Part model, mm, in its own coordinate system. Face numbers are marked on the shaded views. A direction names the side the tool comes from. Round coordinates to 2 decimals unless told otherwise and drop trailing zeros. Loops run counter-clockwise (first coordinate to the right, second up) from the corner with the lowest first, then second, coordinate; pieces in that order, holes last.
(1) Probe probe 1 along Z at (x, y) = (-9, -0.25); probe 2 along Y at (x, z) = (2.5, -7.5); probe 3 along X at (y, z) = (5.5, 7.5) (3 decimals). List the from-to ranges inside material, lowest first.
(2) Tool access for the marked faces 4, 5 and 6: list every direction of +Z, -Z, +X, -X, +Y, -Y with a clear straight run to the whole face (end or side of a thin tool).
(3) Flat gauge pins, fed straight in: pin 1 (1 mm diameter, centred on x = -2, z = -5, fed in from -Y); pin 2 (1.2 mm diameter, centred on x = -9.5, y = 0, fed in from -Z); pin 3 (3 mm diameter, centred on y = 2, z = -13, fed in from -X) (3 decimals). Where does each tip first touch, or does it go through?
(4) Cut at D-D on y = 4. List the corners of the cut face in (x, z) (3 decimals).
(5) Cut at B-B on x = 0. List the corners of the cut face in (y, z), then the cut area to 3 significant figures.
(6) Cut at C-C on z = -3.5. List the corners of the cut face in (x, y) (3 decimals), then the cut area to 3 significant figures.
(7) Mould opens along X. For the marked faces 1, 2 and 3 say: +X half, -X half, draft (parallel to the pull), parting line (faces both ways), or undercut.
(8) Cut at A-A on y = 5.5. List the corners of the cut face in (x, z) (3 decimals), then the cut area to 3 significant figures.
from build123d import *

# Parameters (mm, degrees)
EXTRUDE_1_DEPTH = 1.5
EXTRUDE_2_DEPTH = 3.175
SKETCH_9_R      = 2.3
EXTRUDE_3_DEPTH = 2


with BuildPart() as part:
    # 草图1 → 凸台-拉伸1 (new, symmetric)
    with BuildSketch(Plane(origin=(0, 0, 0), x_dir=(1, 0, 0), z_dir=(0, 1, 0))):
        with BuildLine():
            Line((-13, 2.1), (-13, -2.1))
            ThreePointArc((-13, -2.1), (-12.707106781, -2.807106781), (-12, -3.1))
            Line((-12, -3.1), (-6.4, -3.1))
            ThreePointArc((-6.4, -3.1), (-6.329289322, -3.070710678), (-6.3, -3))
            Line((-6.3, -3), (-6.3, -2.9))
            ThreePointArc((-6.3, -2.9), (-6.270710678, -2.829289322), (-6.2, -2.8))
            Line((-6.2, -2.8), (6.2, -2.8))
            ThreePointArc((6.2, -2.8), (6.270710678, -2.829289322), (6.3, -2.9))
            Line((6.3, -2.9), (6.3, -3))
            ThreePointArc((6.3, -3), (6.329289322, -3.070710678), (6.4, -3.1))
            Line((6.4, -3.1), (12, -3.1))
            ThreePointArc((12, -3.1), (12.707106781, -2.807106781), (13, -2.1))
            Line((13, -2.1), (13, 2.1))
            ThreePointArc((13, 2.1), (12.707106781, 2.807106781), (12, 3.1))
            Line((12, 3.1), (-12, 3.1))
            ThreePointArc((-12, 3.1), (-12.707106781, 2.807106781), (-13, 2.1))
        make_face()
        with BuildLine():
            Line((10.05, 1.65), (8.95, 1.65))
            ThreePointArc((8.95, 1.65), (7.81862915, 1.18137085), (7.35, 0.05))
            Line((7.35, 0.05), (7.35, -0.05))
            ThreePointArc((7.35, -0.05), (7.81862915, -1.18137085), (8.95, -1.65))
            Line((8.95, -1.65), (10.05, -1.65))
            ThreePointArc((10.05, -1.65), (11.18137085, -1.18137085), (11.65, -0.05))
            Line((11.65, -0.05), (11.65, 0.05))
            ThreePointArc((11.65, 0.05), (11.18137085, 1.18137085), (10.05, 1.65))
        make_face(mode=Mode.SUBTRACT)
        with BuildLine():
            Line((-10.05, 1.65), (-8.95, 1.65))
            ThreePointArc((-8.95, 1.65), (-7.81862915, 1.18137085), (-7.35, 0.05))
            Line((-7.35, 0.05), (-7.35, -0.05))
            ThreePointArc((-7.35, -0.05), (-7.81862915, -1.18137085), (-8.95, -1.65))
            Line((-8.95, -1.65), (-10.05, -1.65))
            ThreePointArc((-10.05, -1.65), (-11.18137085, -1.18137085), (-11.65, -0.05))
            Line((-11.65, -0.05), (-11.65, 0.05))
            ThreePointArc((-11.65, 0.05), (-11.18137085, 1.18137085), (-10.05, 1.65))
        make_face(mode=Mode.SUBTRACT)
    extrude(amount=EXTRUDE_1_DEPTH, both=True)

    # 草图8 → 凸台-拉伸2 (add, symmetric)
    with BuildSketch(Plane(origin=(0, 0, 0), x_dir=(0, 0, -1), z_dir=(1, 0, 0))):
        Polygon((6.9, 3), (6.9, 8), (15.9, 8), (15.9, 12.2), (-10.3, 12.2), (-10.3, -1.2), (15.9, -1.2), (15.9, 3), align=None)
    extrude(amount=EXTRUDE_2_DEPTH, both=True)

    # 草图9 → 凸台-拉伸3 (add)
    with BuildSketch(Plane.XY.offset(10.3)):
        with Locations((0, 5.5)):
            Circle(SKETCH_9_R)
    extrude(amount=EXTRUDE_3_DEPTH)


solid = part.part
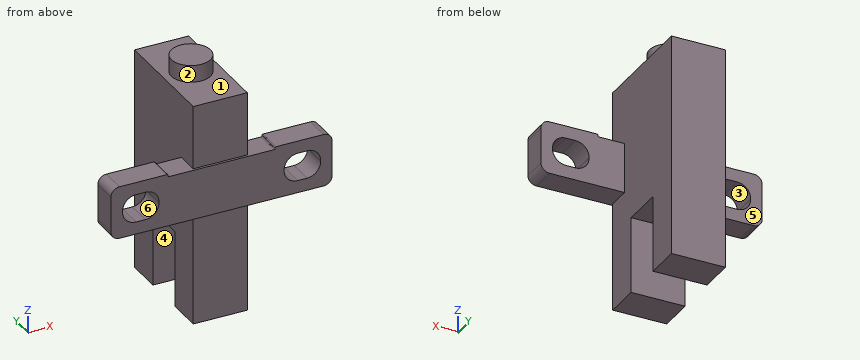
Final values:
1. probe 1: z = -3.1 to -1.65, 1.65 to 3.1
1. probe 2: y = -1.2 to 3, 8 to 12.2
1. probe 3: x = -3.175 to 3.175
2. face 4: -Z, +X, -X
2. face 5: +Z, -Z, -X, +Y
2. face 6: +Y, -Y
3. pin 1: stops at y = -1.2
3. pin 2: stops at z = -3.1
3. pin 3: stops at x = -3.175
4. outline: (-3.175, -6.9) - (3.175, -6.9) - (3.175, 10.3) - (1.744, 10.3) - (1.744, 12.3) - (-1.744, 12.3) - (-1.744, 10.3) - (-3.175, 10.3) - close
5. outline: (-1.5, -3.1) - (-1.2, -3.1) - (-1.2, -15.9) - (3, -15.9) - (3, -6.9) - (8, -6.9) - (8, -15.9) - (12.2, -15.9) - (12.2, 10.3) - (7.8, 10.3) - (7.8, 12.3) - (3.2, 12.3) - (3.2, 10.3) - (-1.2, 10.3) - (-1.2, 2.8) - (-1.5, 2.8) - close
5. area: 317 mm2
6. outline: (-3.175, -1.2) - (3.175, -1.2) - (3.175, 12.2) - (-3.175, 12.2) - close
6. area: 85.1 mm2
7. face 1: draft
7. face 2: parting line
7. face 3: undercut
8. outline: (-3.175, -6.9) - (3.175, -6.9) - (3.175, 10.3) - (2.3, 10.3) - (2.3, 12.3) - (-2.3, 12.3) - (-2.3, 10.3) - (-3.175, 10.3) - close
8. area: 118 mm2
